Input: part model. Units: mm. Frame: model coordinates. Give positions to 0.01 mm unless a question says otherwise; leave off trailing zeros. Loops run counter-clockwise (first coordinate to the right, second up) from the corner with the lowest first, then second, coordinate; pieces in that order, holes last.
from build123d import *

# Parameters (mm, degrees)
SKETCH2_W                        = 252.7
SKETCH2_H                        = 63.5
BOSS_EXTRUDE2_DEPTH              = 12.7
TAP_DRILL_FOR_M8X1_25_TAP1_D     = 6.8
TAP_DRILL_FOR_M8X1_25_TAP1_DEPTH = 40
TAP_DRILL_FOR_M8X1_25_TAP1_TIP   = 2.042926105


with BuildPart() as part:
    # Sketch2 → Boss-Extrude2 (new body)
    with BuildSketch(Plane(origin=(0, 0, 0), x_dir=(1, 0, 0), z_dir=(0, 1, 0))):
        with Locations((-5.813963312, -217.324932993)):
            Rectangle(SKETCH2_W, SKETCH2_H)
    extrude(amount=BOSS_EXTRUDE2_DEPTH)

    # Tap Drill for M8x1.25 Tap1
    with Locations(Plane(origin=(-125.813963312, 12.7, 201.449932993), x_dir=(0, 0, 1), z_dir=(0, 1, 0))):
        with Locations((0, 0), (31.75, 0), (0, 240), (31.75, 240)):
            Hole(TAP_DRILL_FOR_M8X1_25_TAP1_D / 2, depth=TAP_DRILL_FOR_M8X1_25_TAP1_DEPTH)
            with Locations((0, 0, -(TAP_DRILL_FOR_M8X1_25_TAP1_DEPTH + TAP_DRILL_FOR_M8X1_25_TAP1_TIP / 2))):  # 118° drill point
                Cone(0, TAP_DRILL_FOR_M8X1_25_TAP1_D / 2, TAP_DRILL_FOR_M8X1_25_TAP1_TIP, mode=Mode.SUBTRACT)


solid = part.part
(1) Cut plane B-B (z = 234). Return the cut outline in (x, y), and give its area (3 significant figures).
Values follow:
outline: (-132.16, 0) - (-129.12, 0) - (-129.12, 12.7) - (-132.16, 12.7) - close; (-122.51, 0) - (110.88, 0) - (110.88, 12.7) - (-122.51, 12.7) - close; (117.49, 0) - (120.54, 0) - (120.54, 12.7) - (117.49, 12.7) - close
area: 3,040 mm2
(2) Cut plane A-A (z = 202). Return the cut outline in (x, y), and give its area (3 significant figures).
Values follow:
outline: (-132.16, 0) - (-129.17, 0) - (-129.17, 12.7) - (-132.16, 12.7) - close; (-122.46, 0) - (110.83, 0) - (110.83, 12.7) - (-122.46, 12.7) - close; (117.54, 0) - (120.54, 0) - (120.54, 12.7) - (117.54, 12.7) - close
area: 3,040 mm2
(3) Mould query, pull axis X, two halves, no side actions, for faces 1 (the cylindrical face through (112.88, 6.26, 198.31)), 2 (the flat face through (-8, 0, 217)), 3 (the cylindrical face through (-127.12, 6.26, 230.06)), 4 (the flat face through (120.536, 6, 218)). Classes: +X half, -X half, draft (parallel to the pull), parting line (faces both ways), or undercut.
Values follow:
face 1: undercut
face 2: draft
face 3: undercut
face 4: +X half
(4) Ray query, probe 1 along X at (y, z) = (6.5, 232); probe 2 along X at (y, z) = (11.5, 236). Return the intervals inside material, ascending.
Values follow:
probe 1: x = -132.16 to -129, -122.63 to 111, 117.37 to 120.54
probe 2: x = -132.16 to -127.74, -123.89 to 112.26, 116.11 to 120.54
